Source: CAD feature listing. Evaluate the final solid. Frame: model axes, mm. Give positions to 0.01 mm unless a question says otherwise; leave off trailing zeros.
from build123d import *

# Parameters (mm, degrees)
SKETCH1_R           = 1.016
SKETCH1_R_2         = 0.080960088
BOSS_EXTRUDE1_DEPTH = 2.54
SKETCH3_W           = 28
SKETCH3_H           = 11
SKETCH3_W_2         = 10
SKETCH3_H_2         = 28
CUT_EXTRUDE_1_DEPTH = 10
CUT_EXTRUDE2_DEPTH  = 2.54
FILLET_1_R          = 1
BOSS_EXTRUDE2_DEPTH = 0.01


with BuildPart() as part:
    # Sketch1 → Boss-Extrude1 (new body)
    with BuildSketch(Plane(origin=(0, 0, 0), x_dir=(1, 0, 0), z_dir=(0, 1, 0))):
        with BuildLine():
            Line((-23.244816627, 44.45), (23.244816627, 44.45))
            ThreePointArc((23.244816627, 44.45), (24.583514169, 44.270437622), (25.827574029, 43.744444444))
            ThreePointArc((25.827574029, 43.744444444), (35.740062311, 36.101079569), (43.482663438, 26.265909091))
            ThreePointArc((43.482663438, 26.265909091), (45.334600658, 24.468164919), (47.830929781, 23.8125))
            Line((47.830929781, 23.8125), (71.516875, 23.8125))
            Line((71.516875, 23.8125), (76.596875, 18.7325))
            Line((76.596875, 18.7325), (76.596875, -18.7325))
            Line((76.596875, -18.7325), (71.516875, -23.8125))
            Line((71.516875, -23.8125), (47.830929781, -23.8125))
            ThreePointArc((47.830929781, -23.8125), (45.334600658, -24.468164919), (43.482663438, -26.265909091))
            ThreePointArc((43.482663438, -26.265909091), (35.740062311, -36.101079569), (25.827574029, -43.744444444))
            ThreePointArc((25.827574029, -43.744444444), (24.583514169, -44.270437622), (23.244816627, -44.45))
            Line((23.244816627, -44.45), (-23.244816627, -44.45))
            ThreePointArc((-23.244816627, -44.45), (-24.583514169, -44.270437622), (-25.827574029, -43.744444444))
            ThreePointArc((-25.827574029, -43.744444444), (-35.740062311, -36.101079569), (-43.482663438, -26.265909091))
            ThreePointArc((-43.482663438, -26.265909091), (-45.334600658, -24.468164919), (-47.830929781, -23.8125))
            Line((-47.830929781, -23.8125), (-71.516875, -23.8125))
            Line((-71.516875, -23.8125), (-76.596875, -18.7325))
            Line((-76.596875, -18.7325), (-76.596875, 18.7325))
            Line((-76.596875, 18.7325), (-71.516875, 23.8125))
            Line((-71.516875, 23.8125), (-47.830929781, 23.8125))
            ThreePointArc((-47.830929781, 23.8125), (-45.334600658, 24.468164919), (-43.482663438, 26.265909091))
            ThreePointArc((-43.482663438, 26.265909091), (-35.740062311, 36.101079569), (-25.827574029, 43.744444444))
            ThreePointArc((-25.827574029, 43.744444444), (-24.583514169, 44.270437622), (-23.244816627, 44.45))
        make_face()
        with Locations((36.819050096, 28.19800422)):
            Circle(SKETCH1_R, mode=Mode.SUBTRACT)
        with Locations((28.19800422, 36.819050096)):
            Circle(SKETCH1_R, mode=Mode.SUBTRACT)
        with Locations((26.671582547, 26.671582547)):
            Circle(SKETCH1_R_2, mode=Mode.SUBTRACT)
        with Locations((26.671582547, -26.671582547)):
            Circle(SKETCH1_R_2, mode=Mode.SUBTRACT)
        with Locations((36.819050096, -28.19800422)):
            Circle(SKETCH1_R, mode=Mode.SUBTRACT)
        with Locations((28.19800422, -36.819050096)):
            Circle(SKETCH1_R, mode=Mode.SUBTRACT)
        with Locations((-26.671582547, -26.671582547)):
            Circle(SKETCH1_R_2, mode=Mode.SUBTRACT)
        with Locations((-28.19800422, -36.819050096)):
            Circle(SKETCH1_R, mode=Mode.SUBTRACT)
        with Locations((-36.819050096, -28.19800422)):
            Circle(SKETCH1_R, mode=Mode.SUBTRACT)
        with Locations((-26.671582547, 26.671582547)):
            Circle(SKETCH1_R_2, mode=Mode.SUBTRACT)
        with Locations((-36.819050096, 28.19800422)):
            Circle(SKETCH1_R, mode=Mode.SUBTRACT)
        with Locations((-28.19800422, 36.819050096)):
            Circle(SKETCH1_R, mode=Mode.SUBTRACT)
    extrude(amount=BOSS_EXTRUDE1_DEPTH)

    # Sketch3 → 切除-拉伸1 (cut)
    with BuildSketch(Plane(origin=(0, 2.54, 0), x_dir=(1, 0, 0), z_dir=(0, 1, 0))):
        with Locations((0, 28)):
            Rectangle(SKETCH3_W, SKETCH3_H)
        with Locations((0, -28)):
            Rectangle(SKETCH3_W, SKETCH3_H)
        with Locations((-33, 0)):
            Rectangle(SKETCH3_W_2, SKETCH3_H_2)
        with Locations((33, 0)):
            Rectangle(SKETCH3_W_2, SKETCH3_H_2)
    extrude(amount=-CUT_EXTRUDE_1_DEPTH, mode=Mode.SUBTRACT)

    # Sketch4 → Cut-Extrude2 (cut)
    with BuildSketch(Plane(origin=(0, 2.54, 0), x_dir=(1, 0, 0), z_dir=(0, 1, 0))):
        with BuildLine():
            Line((44.592875, 14.605), (67.452875, 14.605))
            ThreePointArc((67.452875, 14.605), (68.350900612, 14.233025612), (68.722875, 13.335))
            Line((68.722875, 13.335), (68.722875, 12.065))
            ThreePointArc((68.722875, 12.065), (68.350900612, 11.166974388), (67.452875, 10.795))
            Line((67.452875, 10.795), (44.592875, 10.795))
            ThreePointArc((44.592875, 10.795), (43.694849388, 11.166974388), (43.322875, 12.065))
            Line((43.322875, 12.065), (43.322875, 13.335))
            ThreePointArc((43.322875, 13.335), (43.694849388, 14.233025612), (44.592875, 14.605))
        make_face()
        with BuildLine():
            Line((68.722875, -13.335), (68.722875, -12.065))
            ThreePointArc((68.722875, -12.065), (68.350900612, -11.166974388), (67.452875, -10.795))
            Line((67.452875, -10.795), (44.592875, -10.795))
            ThreePointArc((44.592875, -10.795), (43.694849388, -11.166974388), (43.322875, -12.065))
            Line((43.322875, -12.065), (43.322875, -13.335))
            ThreePointArc((43.322875, -13.335), (43.694849388, -14.233025612), (44.592875, -14.605))
            Line((44.592875, -14.605), (67.452875, -14.605))
            ThreePointArc((67.452875, -14.605), (68.350900612, -14.233025612), (68.722875, -13.335))
        make_face()
        with BuildLine():
            Line((-44.592875, -14.605), (-67.452875, -14.605))
            ThreePointArc((-67.452875, -14.605), (-68.350900612, -14.233025612), (-68.722875, -13.335))
            Line((-68.722875, -13.335), (-68.722875, -12.065))
            ThreePointArc((-68.722875, -12.065), (-68.350900612, -11.166974388), (-67.452875, -10.795))
            Line((-67.452875, -10.795), (-44.592875, -10.795))
            ThreePointArc((-44.592875, -10.795), (-43.694849388, -11.166974388), (-43.322875, -12.065))
            Line((-43.322875, -12.065), (-43.322875, -13.335))
            ThreePointArc((-43.322875, -13.335), (-43.694849388, -14.233025612), (-44.592875, -14.605))
        make_face()
        with BuildLine():
            Line((-68.722875, 13.335), (-68.722875, 12.065))
            ThreePointArc((-68.722875, 12.065), (-68.350900612, 11.166974388), (-67.452875, 10.795))
            Line((-67.452875, 10.795), (-44.592875, 10.795))
            ThreePointArc((-44.592875, 10.795), (-43.694849388, 11.166974388), (-43.322875, 12.065))
            Line((-43.322875, 12.065), (-43.322875, 13.335))
            ThreePointArc((-43.322875, 13.335), (-43.694849388, 14.233025612), (-44.592875, 14.605))
            Line((-44.592875, 14.605), (-67.452875, 14.605))
            ThreePointArc((-67.452875, 14.605), (-68.350900612, 14.233025612), (-68.722875, 13.335))
        make_face()
    extrude(amount=-CUT_EXTRUDE2_DEPTH, mode=Mode.SUBTRACT)

    # 圆角1
    fillet_1_edges = [part.edges().sort_by_distance(p)[0] for p in [
        (14, 1.27, -33.5),
        (14, 1.27, -22.5),
        (-14, 1.27, -22.5),
        (-14, 1.27, -33.5),
        (14, 1.27, 33.5),
        (-14, 1.27, 33.5),
        (-14, 1.27, 22.5),
        (14, 1.27, 22.5),
        (-28, 1.27, -14),
        (-28, 1.27, 14),
        (-38, 1.27, 14),
        (-38, 1.27, -14),
        (38, 1.27, 14),
        (28, 1.27, 14),
        (28, 1.27, -14),
        (38, 1.27, -14),
    ]]
    fillet(fillet_1_edges, radius=FILLET_1_R)

    # Sketch8 → Boss-Extrude2 (add)
    with BuildSketch(Plane(origin=(0, 2.54, 0), x_dir=(1, 0, 0), z_dir=(0, 1, 0))):
        with BuildLine():
            Line((47.830929781, -23.8125), (71.516875, -23.8125))
            Line((71.516875, -23.8125), (76.596875, -18.7325))
            Line((76.596875, -18.7325), (76.596875, 18.7325))
            Line((76.596875, 18.7325), (71.516875, 23.8125))
            Line((71.516875, 23.8125), (47.830929781, 23.8125))
            ThreePointArc((47.830929781, 23.8125), (45.334600658, 24.468164919), (43.482663438, 26.265909091))
            ThreePointArc((43.482663438, 26.265909091), (35.740062311, 36.101079569), (25.827574029, 43.744444444))
            ThreePointArc((25.827574029, 43.744444444), (24.583514169, 44.270437622), (23.244816627, 44.45))
            Line((23.244816627, 44.45), (-23.244816627, 44.45))
            ThreePointArc((-23.244816627, 44.45), (-24.583514169, 44.270437622), (-25.827574029, 43.744444444))
            ThreePointArc((-25.827574029, 43.744444444), (-35.740062311, 36.101079569), (-43.482663438, 26.265909091))
            ThreePointArc((-43.482663438, 26.265909091), (-45.334600658, 24.468164919), (-47.830929781, 23.8125))
            Line((-47.830929781, 23.8125), (-71.516875, 23.8125))
            Line((-71.516875, 23.8125), (-76.596875, 18.7325))
            Line((-76.596875, 18.7325), (-76.596875, -18.7325))
            Line((-76.596875, -18.7325), (-71.516875, -23.8125))
            Line((-71.516875, -23.8125), (-47.830929781, -23.8125))
            ThreePointArc((-47.830929781, -23.8125), (-45.334600658, -24.468164919), (-43.482663438, -26.265909091))
            ThreePointArc((-43.482663438, -26.265909091), (-35.740062311, -36.101079569), (-25.827574029, -43.744444444))
            ThreePointArc((-25.827574029, -43.744444444), (-24.583514169, -44.270437622), (-23.244816627, -44.45))
            Line((-23.244816627, -44.45), (23.244816627, -44.45))
            ThreePointArc((23.244816627, -44.45), (24.583514169, -44.270437622), (25.827574029, -43.744444444))
            ThreePointArc((25.827574029, -43.744444444), (35.740062311, -36.101079569), (43.482663438, -26.265909091))
            ThreePointArc((43.482663438, -26.265909091), (45.334600658, -24.468164919), (47.830929781, -23.8125))
        make_face()
        with BuildLine():
            Line((47.830929781, -21.5125), (70.564183807, -21.5125))
            Line((70.564183807, -21.5125), (74.296875, -17.779808807))
            Line((74.296875, -17.779808807), (74.296875, 17.779808807))
            Line((74.296875, 17.779808807), (70.564183807, 21.5125))
            Line((70.564183807, 21.5125), (47.830929781, 21.5125))
            ThreePointArc((47.830929781, 21.5125), (44.204372906, 22.465021083), (41.513960172, 25.076704545))
            ThreePointArc((41.513960172, 25.076704545), (34.121909883, 34.466581872), (24.658215363, 41.763888889))
            ThreePointArc((24.658215363, 41.763888889), (23.977410951, 42.051735549), (23.244816627, 42.15))
            Line((23.244816627, 42.15), (-23.244816627, 42.15))
            ThreePointArc((-23.244816627, 42.15), (-23.977410951, 42.051735549), (-24.658215363, 41.763888889))
            ThreePointArc((-24.658215363, 41.763888889), (-34.121909883, 34.466581872), (-41.513960172, 25.076704545))
            ThreePointArc((-41.513960172, 25.076704545), (-44.204372906, 22.465021083), (-47.830929781, 21.5125))
            Line((-47.830929781, 21.5125), (-70.564183807, 21.5125))
            Line((-70.564183807, 21.5125), (-74.296875, 17.779808807))
            Line((-74.296875, 17.779808807), (-74.296875, -17.779808807))
            Line((-74.296875, -17.779808807), (-70.564183807, -21.5125))
            Line((-70.564183807, -21.5125), (-47.830929781, -21.5125))
            ThreePointArc((-47.830929781, -21.5125), (-44.204372906, -22.465021083), (-41.513960172, -25.076704545))
            ThreePointArc((-41.513960172, -25.076704545), (-34.121909883, -34.466581872), (-24.658215363, -41.763888889))
            ThreePointArc((-24.658215363, -41.763888889), (-23.977410951, -42.051735549), (-23.244816627, -42.15))
            Line((-23.244816627, -42.15), (23.244816627, -42.15))
            ThreePointArc((23.244816627, -42.15), (23.977410951, -42.051735549), (24.658215363, -41.763888889))
            ThreePointArc((24.658215363, -41.763888889), (34.121909883, -34.466581872), (41.513960172, -25.076704545))
            ThreePointArc((41.513960172, -25.076704545), (44.204372906, -22.465021083), (47.830929781, -21.5125))
        make_face(mode=Mode.SUBTRACT)
    extrude(amount=BOSS_EXTRUDE2_DEPTH)


solid = part.part
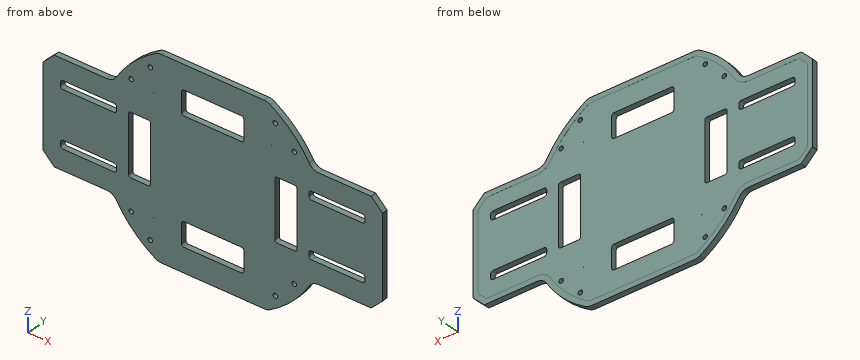
1) Cut plane A-A (x = -50). State how many separate pieces and enclosed holes the cut face has, and give its area (3 significant figures).
Checks:
separate pieces: 3
enclosed holes: 0
area: 102 mm2
2) Contact query for flat-ended pins moving along their axis: P1, Ø2.5, axis at x = 36.82, z = 28.2, coming from the +Y side; P2, Ø1.2, axis at x = 36.82, z = -28.2, coming from the +Y side; P3, Ø1, axis at x = -56, y = 2, coming from the +Z side; P4, Ø1, axis at x = 58.5, y = 0.5, coming from the -Z side. Output: stop coordinate, or through.
Checks:
P1: stops at y = 2.54
P2: passes through
P3: stops at z = 23.81
P4: stops at z = -23.81
3) Ray query, probe 1 along X at (y, z) = (1.3, 7); probe 2 along Z at (x, y) = (-48, 1.8) (1 decimal); probe 3 along Z at (x, y) = (-6.5, 0.1). Return the intervals inside material, ascending.
Checks:
probe 1: x = -76.6 to -38, -28 to 28, 38 to 76.6
probe 2: z = -23.8 to -14.6, -10.8 to 10.8, 14.6 to 23.8
probe 3: z = -44.45 to -33.5, -22.5 to 22.5, 33.5 to 44.45
